```python
from build123d import *

# Parameters (mm, degrees)
CUT_EXTRUDE1_START      = 2
CUT_EXTRUDE1_DEPTH      = 3
FILLET1_R               = 0.25
CUT_EXTRUDE2_DEPTH      = 18.285290042
CUT_EXTRUDE2_DEPTH_BACK = 18.285290042
SKETCH4_W               = 9.25
SKETCH4_H               = 2


with BuildPart() as part:
    # Sketch2 → Revolve1 (revolve)
    with BuildSketch(Plane.XY, mode=Mode.PRIVATE) as revolve1_sk:
        with BuildLine():
            Line((2.5, -16), (2.5, -7.698851501))
            ThreePointArc((2.5, -7.698851501), (1.280768103, -8.115724939), (0, -8.256944444))
            Line((0, -8.256944444), (0, -16))
            Line((0, -16), (2.5, -16))
        make_face()
        with BuildLine():
            Line((2.5, 0), (4.625, 0))
            Line((4.625, 0), (4.625, 1.25))
            ThreePointArc((4.625, 1.25), (2.571630076, 2.907656268), (0, 3.5))
            Line((0, 3.5), (0, -8.256944444))
            ThreePointArc((0, -8.256944444), (1.280768103, -8.115724939), (2.5, -7.698851501))
            Line((2.5, -7.698851501), (2.5, 0))
        make_face()
    revolve(revolve1_sk.sketch.rotate(Axis((0, 21.322324325, 0), (0, -1, 0)), 180), axis=Axis((0, 21.322324325, 0), (0, -1, 0)))

    # Sketch3 → Cut-Extrude1 (cut)
    with BuildSketch(Plane(origin=(0, 0, 0), x_dir=(1, 0, 0), z_dir=(0, 1, 0)).offset(CUT_EXTRUDE1_START)):
        Polygon((2.020725942, 0), (1.010362971, 1.75), (-1.010362971, 1.75), (-2.020725942, 0), (-1.010362971, -1.75), (1.010362971, -1.75), align=None)
    extrude(amount=CUT_EXTRUDE1_DEPTH, mode=Mode.SUBTRACT)

    # Fillet1
    fillet1_edges = [part.edges().sort_by_distance(p)[0] for p in [
        (4.625, 1.25, 0),
        (4.625, 0, 0),
        (2.5, 0, 0),
    ]]
    fillet(fillet1_edges, radius=FILLET1_R)

    # Sketch4 → Cut-Extrude2 (cut, two sides: drawn at the far end of the back side and taken through both)
    with BuildSketch(Plane.XY.offset(-CUT_EXTRUDE2_DEPTH_BACK)):
        with Locations((0, 4)):
            Rectangle(SKETCH4_W, SKETCH4_H)
    extrude(amount=CUT_EXTRUDE2_DEPTH + CUT_EXTRUDE2_DEPTH_BACK, mode=Mode.SUBTRACT)


solid = part.part
```
Geometry check sheet. Reference: the model listing, model coordinates, mm. A direction names the side the tool comes from. Coordinates: 2 decimals unless noted, no trailing zeros. Loops run counter-clockwise (first coordinate to the right, second up) from the corner with the lowest first, then second, coordinate; pieces in that order, holes last. Notation, with made-up numbers: (64.25, 55.25) -> (86.25, 55.25) arc R15 cw to (86.25, 68.25) -> close; hole circle Ø5 at (2.5, 76). An arc over 180 degrees is marked (long way). Put each result on its own line as item: value.
1) Tool access check on faces 5 (the flat face through (1.5, 2.5, -0.9)), 6 (the flat face through (0, 0, 3)), 7 (the flat face through (0, 3, -2)). Record the directions out of +Z, -Z, +X, -X, +Y, -Y that give a thin tool (end or side, any length) a straight path to the whole face; none if there is none.
Result set:
face 5: +Y
face 6: -Y
face 7: +Z, -Z, +X, -X, +Y
2) Gauge pin test, flat ends, axial feed: pin 1 Ø1.5 at (x, y) = (-3, -12) entering from +Z; pin 2 Ø2 at (x, y) = (2.5, -1.5) entering from -Z; pin 3 Ø0.8 at (x, y) = (0, 2.5) entering from +Z. Record the tip position at first contact, or that the pin passes through.
Result set:
pin 1: stops at z = 1.09
pin 2: stops at z = -2
pin 3: stops at z = 3.81
3) Thickness scan on line 1 (X direction, y = -13.25, z = -1.5); line 2 (X direction, y = -10.5, z = -1.25); line 3 (Z direction, x = -1, y = -8.75). Record the ranges inside material, lowest first.
Result set:
line 1: x = -2 to 2
line 2: x = -2.17 to 2.17
line 3: z = -2.29 to 2.29
4) Release check for a two-part mould opening along Z. For faces 1 (the flat face through (0, 2, 0)), 2 (the cylindrical face through (-4.41, 0.71, -1.39)), 3 (the flat face through (0, 2.5, -1.75)), 4 (the flat face through (0, -16, 0)) record: released by +Z, released by -Z, zero draft, split by the parting line, or undercut.
Result set:
face 1: undercut
face 2: split by the parting line
face 3: undercut
face 4: zero draft
5) Cross-section at A-A on y = -10. Record the boundary of the cut face in (x, z), plus the area to 3 significant figures.
Result set:
outline: circle Ø5 at (0, 0)
area: 19.6 mm^2
